Could you check a few things on this model? Use its own coordinates, in mm. A direction names the side the tool comes from. Coordinates: 2 decimals unless noted, no trailing zeros. Loops run counter-clockwise (first coordinate to the right, second up) from the corner with the lowest first, then second, coordinate; pieces in that order, holes last. Notation, with made-up numbers: (47.25, 27.25) -> (53.25, 27.25) arc R22 ccw to (53.25, 59.25) -> close; hole circle Ø4 at (40, 6). An arc over 180 degrees is marked (long way). One line per question, with ' | ' between items. Start each with the question number.
(1) Which directions (+Z, -Z, +X, -X, +Y, -Y) give clear straight access to the entire face, cutting with the end or side of a thin tool? Please do faces 4 (the face through (7.27, 12.49, -0.51)), 5 (the face through (2.12, -4.81, -11.59)), 6 (the face through (7, -13, 3)), 7 (the face through (4, 8, 0)).
(2) Suppose I cut it at D-D (x = 7.75). Please give me the cut outline in (y, z), plus the area to 3 significant figures.
(3) Suppose I cut it at C-C (x = 3). Please give me the cut outline in (y, z).
(4) I'm going to push flat-ended pins straight in: pin 1 Ø4 at (x, y) = (4.5, 5.5) entering from -Z; pin 2 Ø5 at (x, y) = (2.5, 8) entering from +Z; pin 3 Ø1.1 at (x, y) = (7.5, -12.5) entering from +Z; pin 4 Ø1.8 at (x, z) = (3, 0) entering from -Y. Where does each tip first touch, or does it pass through?
(5) If I drill on line 1 along Z through (x, y) = (7.75, 0); line 2 along X through (y, z) = (-9.75, 0); line 3 along X through (y, z) = (-3.5, -5.5), over which ranges is the centre line in solid material (lowest first)?
(6) Suppose I cut it at A-A (z = 0). Please give me the cut outline in (x, y).
(7) If we mould it in two halves opening along Y, with no side actions, what happens to faces 1 (the face through (7.23, 13.49, -0.55)), 2 (the face through (8.5, 12.1, -3.9)), 3 (the face through (6, 3, -3))? For each: pulls with the +Y half, pulls with the -Y half, needs draft (parallel to the pull), parting line crosses it, or undercut.
(8) Suppose I cut it at B-B (y = 0). Please give me the cut outline in (x, z), plus the area to 3 significant figures.
```python
from build123d import *

# Parameters (mm, degrees)
SKETCH_1_R                      = 12.55
EXTRUDE_1_DEPTH                 = 6
SKETCH_2_R                      = 3.2
CUT_EXTRUDE_1_DEPTH             = 6
CUT_EXTRUDE_2_REACH             = 20.735
SKETCH_3_R                      = 1
CUT_EXTRUDE_2_DIRECTION_2_REACH = 20.735
SKETCH_4_R                      = 13.5
EXTRUDE_2_DEPTH                 = 2.5
SKETCH_5_R                      = 12.5
CUT_EXTRUDE_3_DEPTH             = 2.5
FILLET_2_R                      = 2
SKETCH_6_W                      = 2.5
SKETCH_6_H                      = 6
CUT_EXTRUDE_4_DEPTH             = 15


with BuildPart() as part:
    # 草图1 → 凸台-拉伸1 (new body)
    with BuildSketch(Plane(origin=(0, 0, 0), x_dir=(0, 0, -1), z_dir=(1, 0, 0))):
        Circle(SKETCH_1_R)
    extrude(amount=EXTRUDE_1_DEPTH)

    # 草图2 → 切除-拉伸1 (cut)
    with BuildSketch(Plane.ZY):
        Circle(SKETCH_2_R)
    extrude(amount=-CUT_EXTRUDE_1_DEPTH, mode=Mode.SUBTRACT)

    # 草图3 → 切除-拉伸2 (cut, up to next)
    with BuildSketch(Plane(origin=(0, 0, 0), x_dir=(1, 0, 0), z_dir=(0, 1, 0)), mode=Mode.PRIVATE) as cut_extrude_2_sk1:
        with Locations(Location((3, 0, 0), (0, 0, 270))):
            Circle(SKETCH_3_R)
    cut_extrude_2_tool1 = extrude(cut_extrude_2_sk1.sketch, amount=-CUT_EXTRUDE_2_REACH, mode=Mode.PRIVATE) & part.part
    add(cut_extrude_2_tool1.solids().sort_by_distance((3, 0, 0))[0], mode=Mode.SUBTRACT)

    # 草图3 → 切除-拉伸2 direction 2 (cut, up to next)
    with BuildSketch(Plane(origin=(0, 0, 0), x_dir=(1, 0, 0), z_dir=(0, 1, 0)), mode=Mode.PRIVATE) as cut_extrude_2_direction_2_sk1:
        with Locations(Location((3, 0, 0), (0, 0, 270))):
            Circle(SKETCH_3_R)
    cut_extrude_2_direction_2_tool1 = extrude(cut_extrude_2_direction_2_sk1.sketch, amount=CUT_EXTRUDE_2_DIRECTION_2_REACH, mode=Mode.PRIVATE) & part.part
    add(cut_extrude_2_direction_2_tool1.solids().sort_by_distance((3, 0, 0))[0], mode=Mode.SUBTRACT)

    # 草图4 → 凸台-拉伸2 (add)
    with BuildSketch(Plane(origin=(6, 0, 0), x_dir=(0, 0, -1), z_dir=(1, 0, 0))):
        Circle(SKETCH_4_R)
    extrude(amount=EXTRUDE_2_DEPTH)

    # 草图5 → 切除-拉伸3 (cut)
    with BuildSketch(Plane(origin=(8.5, 0, 0), x_dir=(0, 0, -1), z_dir=(1, 0, 0))):
        Circle(SKETCH_5_R)
    extrude(amount=-CUT_EXTRUDE_3_DEPTH, mode=Mode.SUBTRACT)

    # 圆角2
    # the kernel refuses this fillet: 2 mm, written as the material it adds along each edge
    with BuildSketch(Plane(origin=(6, 0, 0), x_dir=(0, 0, -1), z_dir=(0, -1, 0))) as fillet_2_piece_1:
        with BuildLine():
            CenterArc((14.55, -1.702204453), FILLET_2_R, 121.668243254, 58.331756746)
            Line((12.55, -1.702204453), (12.51, -1.702204453))
            Line((12.51, -1.702204453), (12.51, 0))
            Line((12.51, 0), (12.55, 0.04))
            ThreePointArc((12.55, 0.04), (13.025, 0.04), (13.479, 0.034044089))
            Line((13.479, 0.034044089), (13.5, 0))
        make_face()
    revolve(axis=Axis((6, 0, 0), (1, 0, 0)))

    # 草图6 → 切除-拉伸4 (cut)
    with BuildSketch(Plane(origin=(0, 0, 0), x_dir=(1, 0, 0), z_dir=(0, 1, 0))):
        with Locations((7.25, 0)):
            Rectangle(SKETCH_6_W, SKETCH_6_H)
    extrude(amount=-CUT_EXTRUDE_4_DEPTH, mode=Mode.SUBTRACT)


solid = part.part
```
Checks:
1) face 4: +X | face 5: -X | face 6: +X, -Y | face 7: +Y, -Y
2) outline: (-13.16, -3) arc R13.5 ccw (long way) to (-13.16, 3) -> (-12.13, 3) arc R12.5 cw (long way) to (-12.13, -3) -> close | area: 75.6 mm^2
3) outline: (-12.51, -1) arc R12.55 ccw to (12.51, -1) -> (3.04, -1) arc R3.2 cw to (-3.04, -1) -> close; (-12.51, 1) -> (-3.04, 1) arc R3.2 cw to (3.04, 1) -> (12.51, 1) arc R12.55 ccw to start
4) pin 1: stops at z = -12.84 | pin 2: stops at z = 11.28 | pin 3: stops at z = 6.28 | pin 4: passes through
5) line 1: z = -13.5 to -12.5, 12.5 to 13.5 | line 2: x = 0 to 2, 4 to 6 | line 3: x = 0 to 6
6) outline: (0, -12.55) -> (2, -12.55) -> (2, -3.2) -> (0, -3.2) -> close; (0, 3.2) -> (2, 3.2) -> (2, 12.55) -> (0, 12.55) -> close; (4, -12.55) -> (4.3, -12.55) arc R2 cw to (6, -13.5) -> (6, -3.2) -> (4, -3.2) -> close; (4, 3.2) -> (6, 3.2) -> (6, 12.5) -> (8.5, 12.5) -> (8.5, 13.5) -> (6, 13.5) arc R2 cw to (4.3, 12.55) -> (4, 12.55) -> close
7) face 1: parting line crosses it | face 2: needs draft | face 3: undercut
8) outline: (0, -12.55) -> (4.3, -12.55) arc R2 cw to (6, -13.5) -> (8.5, -13.5) -> (8.5, -12.5) -> (6, -12.5) -> (6, -3.2) -> (0, -3.2) -> close; (0, 3.2) -> (6, 3.2) -> (6, 12.5) -> (8.5, 12.5) -> (8.5, 13.5) -> (6, 13.5) arc R2 cw to (4.3, 12.55) -> (0, 12.55) -> close | area: 118 mm^2
